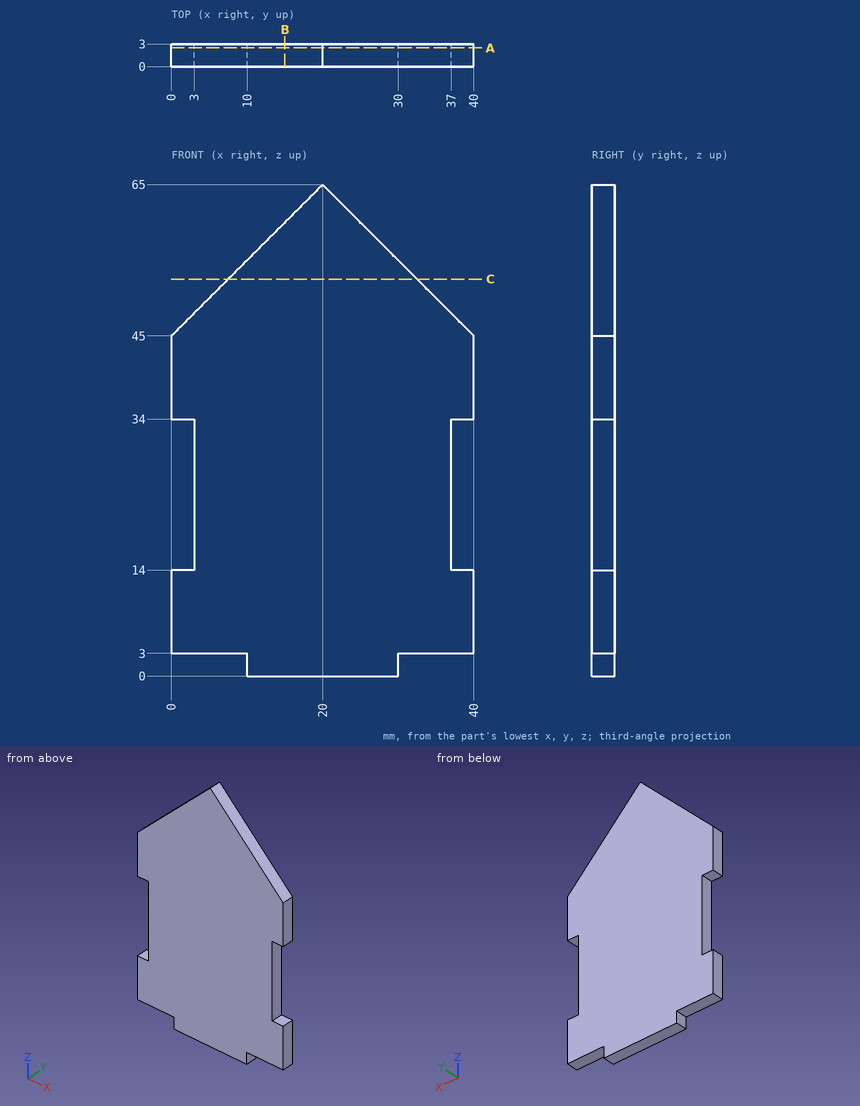
For this review, use the dimensioned drawing (mm, ordinates from the lowest corner) and the shaded views. Give positions to 0.01 mm unless a question says otherwise; leave off trailing zeros. Loops run counter-clockwise (first coordinate to the right, second up) from the corner with the lowest first, then second, coordinate; pieces in that order, holes last. Notation, with made-up numbers: (-16.75, -1) -> (30.25, -1) arc R22 ccw to (30.25, 12) -> close; hole circle Ø2 at (47.5, 27.5). An arc over 180 degrees is marked (long way). One line per question, with ' | ' between items. Start each with the question number.
(1) We need section C-C (z = 52.5). State the section outline as (x, y) points, and give its area (3 significant figures).
(2) For line 1 (X direction, y = 2.75, z = 22.5); line 2 (Z direction, x = 38.5, y = 2.2); line 3 (X direction, y = 1.55, z = 61), list the stretches that pass through material, from the lowest coordinate up.
(3) We need section A-A (y = 2.5). State the section outline as (x, z) points.
(4) We need section B-B (x = 15). State the section outline as (y, z) points.
(5) Insertion check: P1, Ø1.5, axis at x = 1, y = 2, coming from the -Z side; P2, Ø0.9, axis at x = 39, y = 1.5, coming from the +Z side; P3, Ø0.9, axis at y = 1, z = 2, coming from the -X side. Each pin has a flat end and moves straight along its axis. Give the tip position at first contact, or say it passes through.
The answers:
1) outline: (7.5, 0) -> (32.5, 0) -> (32.5, 3) -> (7.5, 3) -> close | area: 75.0 mm^2
2) line 1: x = 3 to 37 | line 2: z = 3 to 14, 34 to 46.5 | line 3: x = 16 to 24
3) outline: (0, 3) -> (10, 3) -> (10, 0) -> (30, 0) -> (30, 3) -> (40, 3) -> (40, 14) -> (37, 14) -> (37, 34) -> (40, 34) -> (40, 45) -> (20, 65) -> (0, 45) -> (0, 34) -> (3, 34) -> (3, 14) -> (0, 14) -> close
4) outline: (0, 0) -> (3, 0) -> (3, 60) -> (0, 60) -> close
5) P1: stops at z = 3 | P2: stops at z = 46.45 | P3: stops at x = 10
